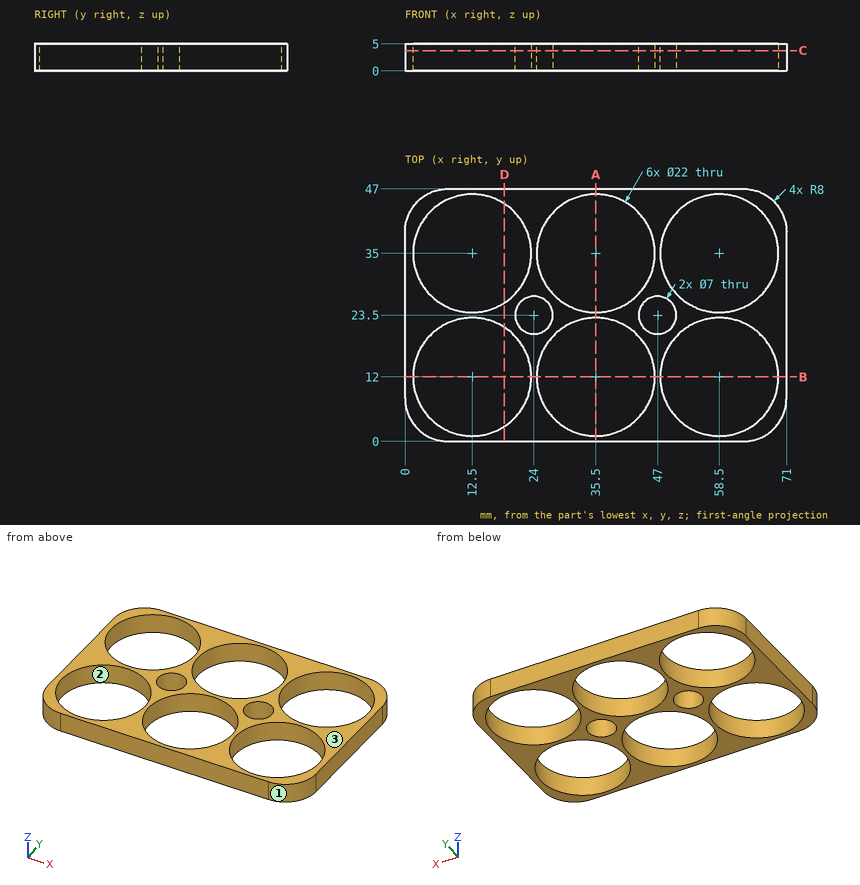
Answer from the drawing. Dimensions are ordinates in mm from the lowest x, y and z of the part. Coordinates: 2 decimals unless noted, no trailing zeros. Write each loop counter-clockwise with the first axis right and the second up, starting at its lowest first coordinate (ties: lowest second). Pieces come first, ordered by that corner, then holes. Notation, with made-up numbers: M 54.25,49.25 L 91.25,49.25 A33 cw 91.25,82.25 Z; hole C 3,-8.5 d5. An arc over 180 degrees is marked long. Use one line per item in the form item = value. Start each with the question number.
1. Each of these flat-tipped pins is pushed along its axis until it touches: P1, Ø4, axis at x = 63, y = 19.5, coming from the -Z side; P2, Ø1, axis at y = 40, z = 1, coming from the +X side. Where does it stop, or does it pass through?
2. The part is cut by section A-A (x = 35.5). Give the vertices of the cut face in (y, z).
3. The part is cut by section C-C (z = 3.75). Give the number of separate pieces and of enclosed holes in the cut face, plus the area to 3 significant figures.
4. The mould has two halves that part along X. Classify the marked faces 1, 2 and 3: released by +X, released by -X, zero draft, split by the parting line, or undercut.
5. The part is cut by section B-B (y = 12). Give the vertices of the cut face in (x, z), plus the area to 3 significant figures.
6. The part is cut by section D-D (x = 18.5). Give the vertices of the cut face in (y, z), plus the area to 3 significant figures.
7. Straight lines are drawn through the part: probe 1 along Y at (x, z) = (12.5, 2.75); probe 2 along X at (y, z) = (16, 1.7); probe 3 along Y at (x, z) = (50, 2.9). For each, find the intervals that lie inside material, in ascending order. Write a range as from..to.
Evaluation:
q1.P1 = through
q1.P2 = 70.98
q2.outline = M 0,0 L 1,0 L 1,5 L 0,5 Z; M 23,0 L 24,0 L 24,5 L 23,5 Z; M 46,0 L 47,0 L 47,5 L 46,5 Z
q3.separate_pieces = 1
q3.enclosed_holes = 8
q3.area = 924 mm^2
q4.face_1 = released by +X
q4.face_2 = undercut
q4.face_3 = zero draft
q5.outline = M 0,0 L 1.5,0 L 1.5,5 L 0,5 Z; M 23.5,0 L 24.5,0 L 24.5,5 L 23.5,5 Z; M 46.5,0 L 47.5,0 L 47.5,5 L 46.5,5 Z; M 69.5,0 L 71,0 L 71,5 L 69.5,5 Z
q5.area = 25.0 mm^2
q6.outline = M 0,0 L 2.78,0 L 2.78,5 L 0,5 Z; M 21.22,0 L 25.78,0 L 25.78,5 L 21.22,5 Z; M 44.22,0 L 47,0 L 47,5 L 44.22,5 Z
q6.area = 50.6 mm^2
q7.probe_1 = 0..1, 23..24, 46..47
q7.probe_2 = 0..2.25, 22.75..25.25, 45.75..48.25, 68.75..71
q7.probe_3 = 0..5.02, 18.98..21.7, 25.3..28.02, 41.98..47
